Autodesk Inventor part; units mm, degrees
ref_plane "YZ Plane" through (0, 0, 0) normal (1, 0, 0) x (0, 1, 0)
ref_plane "XZ Plane" through (0, 0, 0) normal (0, 1, 0) x (-1, 0, 0)
ref_plane "XY Plane" through (0, 0, 0) normal (0, 0, 1) x (1, 0, 0)
sketch "Sketch1" plane through (0, 0, 0) normal (0, 1, 0) x (-1, 0, 0)
  line L0 (-70, 35) -> (70, 35)
  line L1 (75, 30) -> (75, -30)
  line L2 (70, -35) -> (-70, -35)
  line L3 (-75, -30) -> (-75, 30)
  line L4 (-75, 35) -> (75, -35) construction
  line L5 (75, 35) -> (-75, -35) construction
  arc A0 (75, 30) -> (70, 35) centre (70, 30) ccw
  arc A1 (70, -35) -> (75, -30) centre (70, -30) ccw
  arc A2 (-70, 35) -> (-75, 30) centre (-70, 30) ccw
  arc A3 (-75, -30) -> (-70, -35) centre (-70, -30) ccw
  line L6 (-72, 37) -> (72, 37)
  line L7 (77, 32) -> (77, -32)
  line L8 (72, -37) -> (-72, -37)
  line L9 (-77, -32) -> (-77, 32)
  line L10 (-77, 37) -> (77, -37) construction
  line L11 (77, 37) -> (-77, -37) construction
  arc A4 (77, 32) -> (72, 37) centre (72, 32) ccw
  arc A5 (72, -37) -> (77, -32) centre (72, -32) ccw
  arc A6 (-77, -32) -> (-72, -37) centre (-72, -32) ccw
  arc A7 (-72, 37) -> (-77, 32) centre (-72, 32) ccw
  line L12 (74, 39) -> (-74, 39)
  line L13 (-79, 34) -> (-79, -34)
  line L14 (-74, -39) -> (74, -39)
  line L15 (79, -34) -> (79, 34)
  line L16 (79, 39) -> (-79, -39) construction
  line L17 (-79, 39) -> (79, -39) construction
  arc A8 (79, 34) -> (74, 39) centre (74, 34) ccw
  arc A9 (-74, 39) -> (-79, 34) centre (-74, 34) ccw
  arc A10 (-79, -34) -> (-74, -39) centre (-74, -34) ccw
  arc A11 (74, -39) -> (79, -34) centre (74, -34) ccw
  point P0 (0, 0)
  dimension "d0" = 150
  dimension "d1" = 70
  dimension "d2" = 5
  dimension "d6" = 2
  dimension "d7" = 2
  dimension "d8" = 5
  dimension "d9" = 4
  dimension "d10" = 4
  dimension "d11" = 5
extrude "Extrusion1" add sketch "Sketch1" along normal mid plane 15.5 contours L6 A4 L7 A5 L8 A6 L9 A7
extrude "Extrusion2" add sketch "Sketch1" along normal mid plane 19.5 contours A8 L15 A11 L14 A10 L13 A9 L12
properties part number "Box2_walls" material "PPS Plastic"
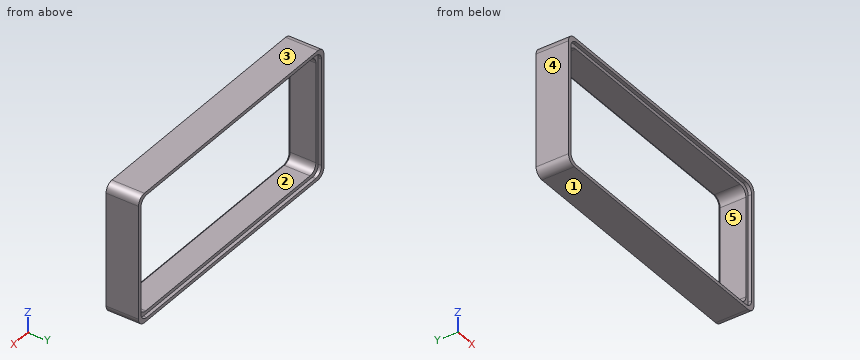
Work out the finished part from the listing and answer in its coordinate system (mm). Face numbers are marked on the shaded views. A direction names the side the tool comes from. Round coordinates to 2 decimals unless told otherwise and drop trailing zeros. Loops run counter-clockwise (first coordinate to the right, second up) from the corner with the lowest first, then second, coordinate; pieces in that order, holes last. Notation, with made-up numbers: M -33.5,0.5 L -10.5,0.5 A37 ccw -10.5,37.5 Z; hole C 85.25,17.5 d10. An arc over 180 degrees is marked long. Use CSV: the item, a comma, the result in double quotes.
Q1. Section B-B, the plane y = -1 is taken. Determine the outline of the cut face in (x, z), then the cut area to 3 significant figures.
Determined:
outline,"M -79,-34 A5 ccw -74,-39 L 74,-39 A5 ccw 79,-34 L 79,34 A5 ccw 74,39 L -74,39 A5 ccw -79,34 Z; hole M -75,-30 A5 ccw -70,-35 L 70,-35 A5 ccw 75,-30 L 75,30 A5 ccw 70,35 L -70,35 A5 ccw -75,30 Z"
area,"1,820 mm2"
Q2. A tool of negligible diameter and unlimited length cuts with its end or side. For the marked faces 4 and 5, from which of +Z, -Z, +X, -X, +Y, -Y can it reach the whole face along a straight path? Write none if from no direction.
Determined:
face 4,"+Z, -Z, -X, +Y, -Y"
face 5,"+Y, -Y"
Q3. Section A-A, the plane x = 20 is taken. Determine the outline of the cut face in (y, z), then the cut area to 3 significant figures.
Determined:
outline,"M -9.75,-39 L 9.75,-39 L 9.75,-37 L 7.75,-37 L 7.75,-35 L -7.75,-35 L -7.75,-37 L -9.75,-37 Z; M -9.75,37 L -7.75,37 L -7.75,35 L 7.75,35 L 7.75,37 L 9.75,37 L 9.75,39 L -9.75,39 Z"
area,"140 mm2"
Q4. The mould has two halves that part along Z. Classify the marked faces 1, 2 and 3: pulls with the +Z half, pulls with the -Z half, needs draft (parallel to the pull), parting line crosses it, or undercut.
Determined:
face 1,"pulls with the -Z half"
face 2,"undercut"
face 3,"pulls with the +Z half"
Q5. Consider L1, parallel to X at y = -7.5, z = -30; L2, parallel to Z at x = 56, y = 4.25; L3, parallel to X at y = 8.5, z = 20. Determine where each line is inside the solid, lowest interval first.
Determined:
L1,"-79 to -75, 75 to 79"
L2,"-39 to -35, 35 to 39"
L3,"-79 to -77, 77 to 79"
Q6. Section C-C, the plane z = 18 is taken. Determine the outline of the cut face in (x, y).
Determined:
outline,"M -79,-9.75 L -77,-9.75 L -77,-7.75 L -75,-7.75 L -75,7.75 L -77,7.75 L -77,9.75 L -79,9.75 Z; M 75,-7.75 L 77,-7.75 L 77,-9.75 L 79,-9.75 L 79,9.75 L 77,9.75 L 77,7.75 L 75,7.75 Z"
